Could you check a few things on this drawing? It's one solid part, dimensions in mm from its lowest x, y, z. A direction names the side the tool comes from. Coordinates: 2 decimals unless noted, no trailing zeros. Order: outer loops, then holes, each group sorted by start corner. A loop starts at its lowest first (then second) coordinate and runs counter-clockwise, first axis right, second up.
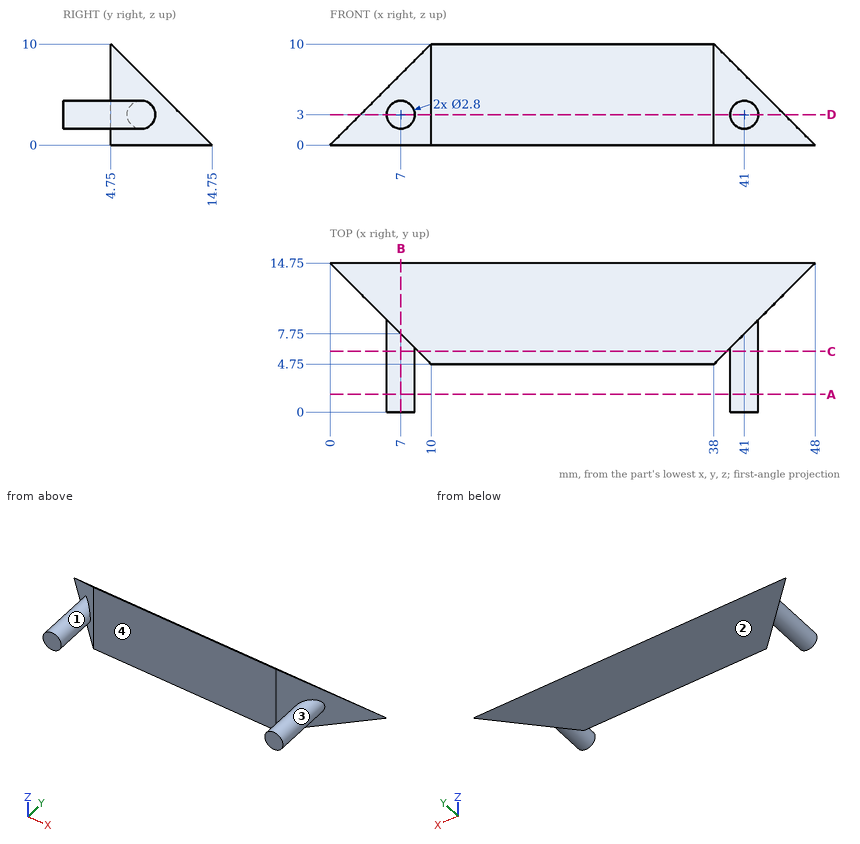
Item 1: Suppose I cut it at B-B (x = 7). List the corners of the cut face in (y, z) for me, and give its area (3 significant figures).
Item 2: For pin 1 Ø8 at (x, y) = (22.5, 2.5) entering from +Z; pin 2 Ø3 at (y, z) = (7.5, 3.5) entering from +X; pin 3 Ø1.5 at (x, y) = (37, 10) entering from +Z; pin 4 Ø2 at (x, z) = (7.5, 1.5) entering from +Y, each with a flat end and sliding along its axis, tell me the tip position at first contact or that it passes through.
Item 3: Thinking about a two-plate mould opening in X: for the marked faces 1 and 2, which applies, +X half, -X half, draft (parallel to the pull), parting line (faces both ways), or undercut?
Item 4: Suppose I cut it at A-A (y = 1.75). List the corners of the cut face in (x, z) for me.
Item 5: Suppose I cut it at D-D (z = 3). List the corners of the cut face in (x, y) for me.
Item 6: Suppose I cut it at C-C (y = 6). List the corners of the cut face in (x, z) for me, and give its area (3 significant figures).
Item 7: Which directions (+Z, -Z, +X, -X, +Y, -Y) give clear straight access to the entire face, cutting with the end or side of a thin tool? Please do the marked faces 3 and 4.
Item 8: I need wall thicknesses on line 1 (Y direction, x = 21, z = 4.75); line 2 (Y direction, x = 31, z = 6.5); line 3 (X direction, y = 9.5, z = 4.75). Which ranges of each line are inside material? Lowest first, please.
Geometry results:
1. outline: (0, 1.6) - (7.75, 1.6) - (7.75, 0) - (14.75, 0) - (7.75, 7) - (7.75, 4.4) - (0, 4.4) - close
1. area: 46.2 mm2
2. pin 1: stops at z = 10
2. pin 2: stops at x = 42.4
2. pin 3: stops at z = 5.5
2. pin 4: stops at y = 14.25
3. face 1: undercut
3. face 2: draft
4. outline: circle Ø2.8 at (7, 3); circle Ø2.8 at (41, 3)
5. outline: (3, 11.75) - (5.6, 9.15) - (5.6, 0) - (8.4, 0) - (8.4, 6.35) - (10, 4.75) - (38, 4.75) - (39.6, 6.35) - (39.6, 0) - (42.4, 0) - (42.4, 9.15) - (45, 11.75) - close
6. outline: circle Ø2.8 at (7, 3); (8.75, 0) - (39.25, 0) - (39.25, 8.75) - (8.75, 8.75) - close; circle Ø2.8 at (41, 3)
6. area: 279 mm2
7. face 3: -Y
7. face 4: +Z, -Z, -Y
8. line 1: y = 4.75 to 10
8. line 2: y = 4.75 to 8.25
8. line 3: x = 5.25 to 42.75
